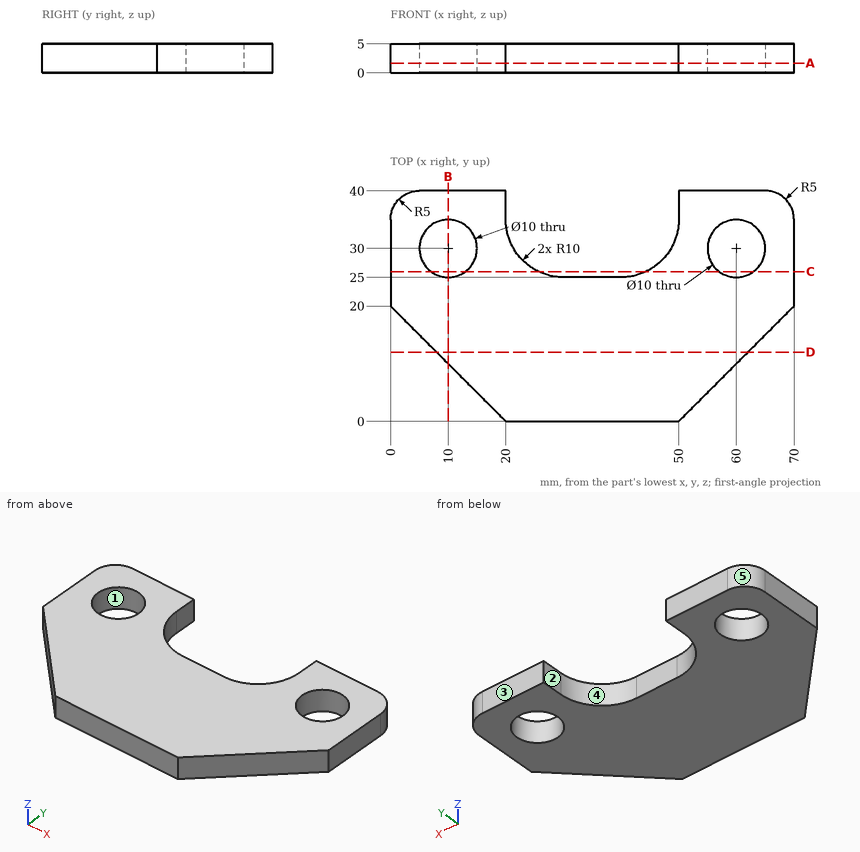
Geometry check sheet. Reference: drawing and pictorial views, mm from the part's lowest x, y, z. A direction names the side the tool comes from. Give positions to 0.01 mm unless a question says otherwise; leave off trailing zeros. Order: outer loops, then holes, each group sorted by start corner. A loop starts at its lowest first (then second) coordinate and runs counter-clockwise, first axis right, second up. Notation, with made-up numbers: M 82.5,13.25 L 138.5,13.25 A36 ccw 138.5,47.25 Z; hole C 26,69 d4. An arc over 180 degrees is marked long. Answer in a Markdown table with one row per item. Add a question column.
Item 1: Section check C-C, the plane y = 26. Enter the section's corners in (x, z), and give its area (3 significant figures).
Item 2: Section check B-B, the plane x = 10. Enter the section's corners in (y, z).
Item 3: Section check D-D, the plane y = 12. Enter the section's corners in (x, z), and give its area (3 significant figures).
Item 4: Mould release check, pull along X, two halves, no side actions. Record for the marked faces 3, 4 and 5: released by +X, released by -X, zero draft, split by the parting line, or undercut.
Item 5: Scan lines: probe 1 along X at (y, z) = (31.5, 1.3); probe 2 along X at (y, z) = (34, 2.4); probe 3 along Y at (x, z) = (37, 4.8). Record each from-to range of solid material in increasing order. Write a range as from..to.
Item 6: Tool access check on the marked faces 1 and 2. Record the directions out of +Z, -Z, +X, -X, +Y, -Y that give a thin tool (end or side, any length) a straight path to the whole face; none if there is none.
Item 7: Gauge pin test, flat ends, axial feed: pin 1 (2 mm diameter, centred on x = 22.5, z = 2, fed in from +Y); pin 2 (2.5 mm diameter, centred on y = 37, z = 3, fed in from -X). Record the tip position at first contact, or that the pin passes through.
Item 8: Section check A-A, the plane z = 1.7. Enter the section's corners in (x, y), and give its area (3 significant figures).
Filled sheet:
| question | item | result |
|---|---|---|
| 1 | outline | M 0,0 L 7,0 L 7,5 L 0,5 Z; M 13,0 L 25.64,0 L 25.64,5 L 13,5 Z; M 44.36,0 L 57,0 L 57,5 L 44.36,5 Z; M 63,0 L 70,0 L 70,5 L 63,5 Z |
| 1 | area | 196 mm^2 |
| 2 | outline | M 10,0 L 25,0 L 25,5 L 10,5 Z; M 35,0 L 40,0 L 40,5 L 35,5 Z |
| 3 | outline | M 8,0 L 62,0 L 62,5 L 8,5 Z |
| 3 | area | 270 mm^2 |
| 4 | face 3 | zero draft |
| 4 | face 4 | undercut |
| 4 | face 5 | released by -X |
| 5 | probe 1 | x = 0..5.23, 14.77..20.63, 49.37..55.23, 64.77..70 |
| 5 | probe 2 | x = 0..7, 13..20.05, 49.95..57, 63..70 |
| 5 | probe 3 | y = 0..25 |
| 6 | face 1 | +Z, -Z |
| 6 | face 2 | +Z, -Z, +Y |
| 7 | pin 1 | stops at y = 29.73 |
| 7 | pin 2 | stops at x = 0.06 |
| 8 | outline | M 0,20 L 20,0 L 50,0 L 70,20 L 70,35 A5 ccw 65,40 L 50,40 L 50,35 A10 cw 40,25 L 30,25 A10 cw 20,35 L 20,40 L 5,40 A5 ccw 0,35 Z; hole C 10,30 d10; hole C 60,30 d10 |
| 8 | area | 1,830 mm^2 |
